Model file for the job. Use its own axes, mm. A direction names the side the tool comes from. Give positions to 0.01 mm unless a question says otherwise; leave off trailing zeros. Order: outer loops, then holes, each group sorted by start corner. A loop starts at its lowest first (then second) coordinate and runs counter-clockwise, first axis right, second up. Notation, with made-up numbers: (-27.75, 77) -> (-2.75, 77) arc R20 cw to (-2.75, 105) -> close; hole circle Ø7 at (44, 25.25). An arc over 180 degrees is marked (long way). Answer in a Markdown table with one row per item. Add a question column.
from build123d import *

# Parameters (mm, degrees)
F1_DEPTH = 19.05
F2_R     = 3.81
F3_DEPTH = 25.4


with BuildPart() as f1:
    # F0 (on Front) → F1 (new body)
    with BuildSketch(Plane.XZ):
        with BuildLine():
            Line((10.16, 7.7975), (10.16, 25.4))
            Line((10.16, 25.4), (-10.16, 25.4))
            Line((-10.16, 25.4), (-10.16, -25.4))
            Line((-10.16, -25.4), (10.16, -25.4))
            Line((10.16, -25.4), (10.16, -7.7975))
            Line((10.16, -7.7975), (7.334133, -7.7975))
            Line((7.334133, -7.7975), (7.334133, -5.3975))
            ThreePointArc((7.334133, -5.3975), (4.067502, 0.000618), (7.335229, 5.398074))
            Line((7.335229, 5.398074), (7.335229, 7.7975))
            Line((7.335229, 7.7975), (10.16, 7.7975))
        make_face()
    extrude(amount=F1_DEPTH)

    # F2 (on face) → F3 (cut)
    with BuildSketch(Plane(origin=(-10.16, 0, 0), x_dir=(0, -1, 0), z_dir=(-1, 0, 0))):
        with Locations((9.525, 17.018)):
            Circle(F2_R)
        with Locations((9.525, -17.018)):
            Circle(F2_R)
    extrude(amount=-F3_DEPTH, mode=Mode.SUBTRACT)


solid = f1.part
Item 1: Saw through at A-A on y = -9.25. List the corners of the cut face in (x, z) (1 decimal), plus the area to 3 significant figures.
Item 2: Which spindle directions (+Z, -Z, +X, -X, +Y, -Y) get a long thin tool onto all of the face, cutting with end or side? Do faces 1 (the flat face through (7.334, -9, -7)), 2 (the flat face through (10.16, -9, 13)). Say none if no direction does.
Item 3: Saw through at D-D on y = -14.5. List the corners of the cut face in (x, z) (1 decimal).
Item 4: Saw through at B-B on z = 14.5. List the corners of the cut face in (x, y), plus the area to 3 significant figures.
Item 5: Wall check: line 1 (Z direction, x = -7, y = -11.25); line 2 (Z direction, x = 6.5, y = -10.75); line 3 (Z direction, x = 5, y = -5.25). Give the ranges that are in metal, low to high.
Item 6: Saw through at C-C on x = 5. List the corners of the cut face in (y, z) (3 decimals), plus the area to 3 significant figures.
Item 7: Two-plate mould, pull along Y, no slides. Class faces 3 (the flat face through (-10.16, -9, 0)), 4 (the cylindrical face through (-0.14, -6.72, -14.44)), 5 (the flat face through (0, 0, 0)), 6 (the flat face through (0, -19.05, 0)): pulls with the +Y half, pulls with the -Y half, needs draft (parallel to the pull), parting line crosses it, or undercut.
Evaluation:
| question | item | result |
|---|---|---|
| 1 | outline | (-10.2, -25.4) -> (10.2, -25.4) -> (10.2, -20.8) -> (-10.2, -20.8) -> close; (-10.2, -13.2) -> (10.2, -13.2) -> (10.2, -7.8) -> (7.3, -7.8) -> (7.3, -5.4) arc R6.1 cw to (7.3, 5.4) -> (7.3, 7.8) -> (10.2, 7.8) -> (10.2, 13.2) -> (-10.2, 13.2) -> close; (-10.2, 20.8) -> (10.2, 20.8) -> (10.2, 25.4) -> (-10.2, 25.4) -> close |
| 1 | area | 654 mm2 |
| 2 | face 1 | +X, +Y, -Y |
| 2 | face 2 | +Z, -Z, +X, +Y, -Y |
| 3 | outline | (-10.2, -25.4) -> (10.2, -25.4) -> (10.2, -7.8) -> (7.3, -7.8) -> (7.3, -5.4) arc R6.1 cw to (7.3, 5.4) -> (7.3, 7.8) -> (10.2, 7.8) -> (10.2, 25.4) -> (-10.2, 25.4) -> close |
| 4 | outline | (-10.16, -19.05) -> (10.16, -19.05) -> (10.16, -12.38) -> (-10.16, -12.38) -> close; (-10.16, -6.67) -> (10.16, -6.67) -> (10.16, 0) -> (-10.16, 0) -> close |
| 4 | area | 271 mm2 |
| 5 | line 1 | z = -25.4 to -20.42, -13.62 to 13.62, 20.42 to 25.4 |
| 5 | line 2 | z = -25.4 to -20.63, -13.41 to -4.87, 4.87 to 13.41, 20.63 to 25.4 |
| 5 | line 3 | z = -25.4 to -3.24, 3.24 to 25.4 |
| 6 | outline | (-19.05, -25.4) -> (0, -25.4) -> (0, -3.239) -> (-19.05, -3.239) -> close; (-19.05, 3.239) -> (0, 3.239) -> (0, 25.4) -> (-19.05, 25.4) -> close; hole circle Ø7.62 at (-9.525, -17.018); hole circle Ø7.62 at (-9.525, 17.018) |
| 6 | area | 753 mm2 |
| 7 | face 3 | needs draft |
| 7 | face 4 | undercut |
| 7 | face 5 | pulls with the +Y half |
| 7 | face 6 | pulls with the -Y half |
